Work out the finished part from the listing and answer in its coordinate system (mm). Face numbers are marked on the shaded views. Coordinates: 2 decimals unless noted, no trailing zeros. Order: outer loops, then holes, each group sorted by start corner. A loop starts at its lowest first (then second) coordinate and runs counter-clockwise, first axis right, second up.
1. The part is cut by section B-B, the plane z = 0. Give the vertices of the cut face in (x, y).
2. The part is cut by section D-D, the plane y = -1.25. Give the vertices of the cut face in (x, z), then the cut area to 3 significant figures.
3. Flat-ended cylindrical pins translate along their axes: pin 1 Ø8 at (x, z) = (15, 20.5) entering from +Y; pin 2 Ø4 at (x, y) = (18.5, -8) entering from +Z; pin 3 Ø1.5 at (x, y) = (-13.5, -3) entering from +Z; pin 4 Ø12 at (x, y) = (4, -14.5) entering from -Z. Find the tip coordinate at first contact, or state that the pin passes through.
4. The part is cut by section C-C, the plane y = -18.5. Give the vertices of the cut face in (x, z).
5. The part is cut by section A-A, the plane x = 0. Give the vertices of the cut face in (y, z), then the cut area to 3 significant figures.
6. Find the intervals of material crossed by probe 1 along Z at (x, y) = (0, -12); probe 2 along Y at (x, z) = (-22.5, 9.5); probe 3 along X at (y, z) = (-14.5, 25), in increasing order.
7. Determine the mould class of the marked faces 1, 2 and 3 for opening direction X: +X half, -X half, draft (parallel to the pull), parting line (faces both ways), or undercut.
```python
from build123d import *

# Parameters (mm, degrees)
F0_R     = 35
F1_DEPTH = 21
F2_R     = 30
F3_DEPTH = 17
F4_R     = 35
F4_R_2   = 32.5
F5_DEPTH = 4


with BuildPart() as f1:
    # F0 (on Front) → F1 (new body)
    with BuildSketch(Plane.XZ):
        Circle(F0_R)
    extrude(amount=F1_DEPTH)

    # F2 (on face) → F3 (cut)
    with BuildSketch(Plane.XZ.offset(21)):
        Circle(F2_R)
    extrude(amount=-F3_DEPTH, mode=Mode.SUBTRACT)

    # F4 (on face) → F5 (cut)
    with BuildSketch(Plane.XZ.offset(21)):
        Circle(F4_R)
        Circle(F4_R_2, mode=Mode.SUBTRACT)
    extrude(amount=-F5_DEPTH, mode=Mode.SUBTRACT)


solid = f1.part
```
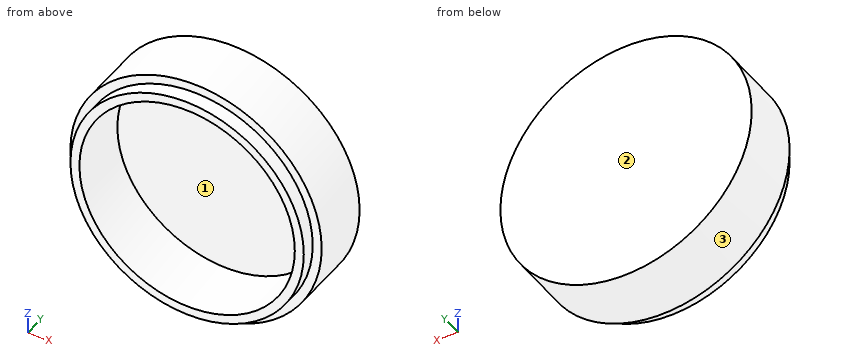
Geometry says:
1. outline: (-35, -17) - (-32.5, -17) - (-32.5, -21) - (-30, -21) - (-30, -4) - (30, -4) - (30, -21) - (32.5, -21) - (32.5, -17) - (35, -17) - (35, 0) - (-35, 0) - close
2. outline: circle Ø70 at (0, 0)
2. area: 3,850 mm2
3. pin 1: stops at y = 0
3. pin 2: stops at z = 30.87
3. pin 3: stops at z = 32.6
3. pin 4: stops at z = -35
4. outline: circle Ø65 at (0, 0); hole circle Ø60 at (0, 0)
5. outline: (-21, -32.5) - (-17, -32.5) - (-17, -35) - (0, -35) - (0, 35) - (-17, 35) - (-17, 32.5) - (-21, 32.5) - (-21, 30) - (-4, 30) - (-4, -30) - (-21, -30) - close
5. area: 430 mm2
6. probe 1: z = -35 to -30, 30 to 35
6. probe 2: y = -4 to 0
6. probe 3: x = -24.49 to -16.58, 16.58 to 24.49
7. face 1: undercut
7. face 2: draft
7. face 3: parting line
